Could you check a few things on this drawing? It's one solid part, dimensions in mm from its lowest x, y, z. Give positions to 0.01 mm unless a question says otherwise; leave off trailing zeros. Loops run counter-clockwise (first coordinate to the right, second up) from the corner with the lowest first, then second, coordinate; pieces in that order, holes last.
1. For P1, Ø1, axis at y = 1.5, z = 1, coming from the -X side; P2, Ø2.5, axis at x = 5, z = 9, coming from the +Y side, each with a flat end and sliding along its axis, tell me the tip position at first contact or that it passes through.
2. Imagine slicing it at D-D (z = 12). List the corners of the cut face in (x, y) for me, plus the area to 3 significant figures.
3. I need wall thicknesses on line 1 along X through (y, z) = (0.95, 9); line 2 along Z through (x, y) = (45, 1.5); line 3 along X through (y, z) = (1.95, 10). Which ranges of each line are inside material? Lowest first, please.
4. Imagine slicing it at A-A (y = 1.85). List the corners of the cut face in (x, z) for me.
5. Thinking about a two-plate mould opening in X: for the marked faces 1, 2, 3 and 4, which applies, +X half, -X half, draft (parallel to the pull), parting line (faces both ways), or undercut?
6. Imagine slicing it at C-C (z = 8.5). List the corners of the cut face in (x, y) for me, plus the area to 3 significant figures.
7. Imagine slicing it at B-B (x = 44). List the corners of the cut face in (y, z) for me.
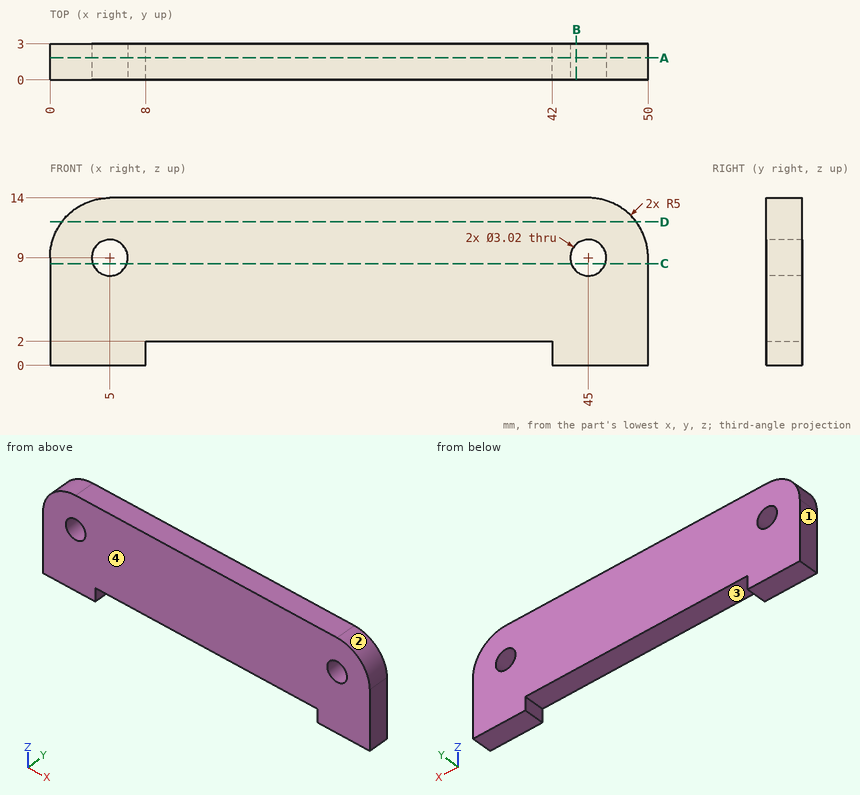
Derived:
1. P1: stops at x = 0
1. P2: passes through
2. outline: (1, 0) - (49, 0) - (49, 3) - (1, 3) - close
2. area: 144 mm2
3. line 1: x = 0 to 3.49, 6.51 to 43.49, 46.51 to 50
3. line 2: z = 0 to 7.49, 10.51 to 14
3. line 3: x = 0.1 to 3.87, 6.13 to 43.87, 46.13 to 49.9
4. outline: (0, 0) - (8, 0) - (8, 2) - (42, 2) - (42, 0) - (50, 0) - (50, 9) arc R5 ccw to (45, 14) - (5, 14) arc R5 ccw to (0, 9) - close; hole circle Ø3.02 at (5, 9); hole circle Ø3.02 at (45, 9)
5. face 1: -X half
5. face 2: +X half
5. face 3: undercut
5. face 4: draft
6. outline: (0, 0) - (3.58, 0) - (3.58, 3) - (0, 3) - close; (6.42, 0) - (43.58, 0) - (43.58, 3) - (6.42, 3) - close; (46.42, 0) - (50, 0) - (50, 3) - (46.42, 3) - close
6. area: 133 mm2
7. outline: (0, 0) - (3, 0) - (3, 7.87) - (0, 7.87) - close; (0, 10.13) - (3, 10.13) - (3, 14) - (0, 14) - close
